Work out the finished part from the listing and answer in its coordinate system (mm). Give positions to 0.01 mm unless a question says otherwise; leave off trailing zeros. Loops run counter-clockwise (first coordinate to the right, second up) from the corner with the lowest first, then second, coordinate; pieces in that order, holes last. Notation, with made-up numbers: (75, -1.75) - (133, -1.75) arc R24 ccw to (133, 20.25) - close; hole circle Ø4 at (85.5, 84.5). An arc over 180 degrees is marked (long way). Use CSV: the item, a comma, the result in double quotes.
from build123d import *

# Parameters (mm, degrees)
F0_R      = 13.478369
F1_DEPTH  = 55.372
F2_SIZE   = 5.08
F1_FACE_R = 13.478369
F3_DEPTH  = 25.4


with BuildPart() as f1:
    # F0 (on Front) → F1 (new body)
    with BuildSketch(Plane.XZ):
        with Locations((-22.897817, -2.051539)):
            Circle(F0_R)
    extrude(amount=-F1_DEPTH)

    # F2
    f2_edges = [f1.edges().sort_by_distance(p)[0] for p in [
        (-36.376187, 0, -2.051539),
    ]]
    chamfer(f2_edges, length=F2_SIZE)

    # F1_face (on face) → F3 (join)
    with BuildSketch(Plane(origin=(-22.897817, 55.372, -2.051539), x_dir=(1, 0, 0), z_dir=(0, 1, 0))):
        Circle(F1_FACE_R)
    extrude(amount=F3_DEPTH)


solid = f1.part
Item 1: Given P1, Ø2, axis at y = 58, z = 8, coming from the +X side; P2, Ø10, axis at y = 44, z = 6.5, coming from the -X side; P3, Ø10, axis at x = -29, y = 28.5, coming from the -Z side, each flat-ended and moving along its own axis, determine where each tip first touches the part or whether it passes through.
Determined:
P1,"stops at x = -12.91"
P2,"stops at x = -35.9"
P3,"stops at z = -15.48"
Item 2: Find the intervals of material crossed by line 1 (Z direction, x = -22.75, y = 52.5); line 2 (X direction, y = 23, z = -10.75); line 3 (Y direction, x = -21, z = 7), in increasing order.
Determined:
line 1,"z = -15.53 to 11.43"
line 2,"x = -33.19 to -12.6"
line 3,"y = 0.85 to 80.77"
Item 3: A cutting plane is placed at A-A on y = 67.5. Determine the outline of the cut face in (x, z), and give its area (3 significant figures).
Determined:
outline,"circle Ø26.96 at (-22.9, -2.05)"
area,"571 mm²"
